Check sheet for the modelled part. Datum: model origin and axes. Units: mm. Face numbers are marked on the shaded views. A direction names the side the tool comes from. Give positions to 0.01 mm unless a question says otherwise; leave off trailing zeros. Write each loop counter-clockwise with the first axis right and the second up, starting at its lowest first coordinate (ties: lowest second). Pieces come first, ordered by that corner, then holes. Notation, with made-up numbers: M 22.25,63 L 30.25,63 A28 ccw 30.25,84 Z; hole C -36,35 d4. An arc over 180 degrees is marked long. Write item = value, one per line. Start each with the question number.
1) Sectioned sample at B-B, the plane x = 0. Record the cut outline in (y, z).
2) Draft check along Z on the marked faces 6, 7, 8 and 9. Enter one of: pulls with the +Z half, pulls with the -Z half, needs draft (parallel to the pull), parting line crosses it, or undercut.
3) Set-up check for the marked faces 1, 2, 3, 4 and 5: record each of +Z, -Z, +X, -X, +Y, -Y from which the full face is reachable in a straight line by a thin tool's end or side.
4) Gauge pin test, flat ends, axial feed: pin 1 (4.5 mm diameter, centred on y = -9.5, z = 89.5, fed in from -X); pin 2 (1.3 mm diameter, centred on y = 8.5, z = 89.5, fed in from +X); pin 3 (3 mm diameter, centred on y = 6.5, z = 90.5, fed in from +X). Record the tip position at first contact, or that the pin passes through.
5) Scan lines: L1, parallel to Y at x = -5.1, z = 92.5; L2, parallel to X at y = -10, z = 92.25; L3, parallel to Y at x = 0.5, z = 95. Record each from-to range of solid material in increasing order.
6) Sectioned sample at A-A, the plane y = 8. Record the cut outline in (x, z).
7) Sectioned sample at C-C, the plane z = 92.5. Count the separate pieces of the cut face and the enclosed holes in it, then the cut area to 3 significant figures.
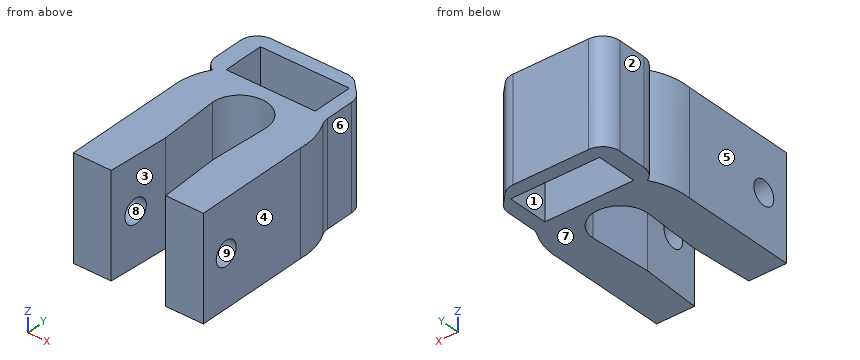
from build123d import *

# Parameters (mm, degrees)
CLIP_DEPTH          = 15
SKETCH7_R           = 1.75
CUT_EXTRUDE4_DEPTH  = 19.812
SKETCH8_W           = 17.539999972
SKETCH8_H           = 9.000000002
BOSS_EXTRUDE1_DEPTH = 15
SKETCH10_W          = 13
SKETCH10_H          = 6
CUT_EXTRUDE5_DEPTH  = 15
CHAMFER2_SIZE       = 3
FILLET1_R           = 2.5


with BuildPart() as part:
    # Sketch1 → Clip (new body)
    with BuildSketch(Plane(origin=(0, -100, 100), x_dir=(1, 0, 0), z_dir=(0, 0, -1))):
        with BuildLine():
            Line((-3.447825682, -91.120916541), (-3.96875, -100))
            ThreePointArc((-3.96875, -100), (0, -103.96875), (3.96875, -100))
            Line((3.96875, -100), (3.447825682, -91.120916541))
            Line((3.447825682, -91.120916541), (3.96875, -82.230916541))
            Line((3.96875, -82.230916541), (9.496072463, -82.230916541))
            Line((9.496072463, -82.230916541), (9.496072463, -99.258223228))
            ThreePointArc((9.496072463, -99.258223228), (0, -109.525), (-9.496072463, -99.258223228))
            Line((-9.496072463, -99.258223228), (-9.496072463, -82.230916541))
            Line((-9.496072463, -82.230916541), (-3.96875, -82.230916541))
            Line((-3.96875, -82.230916541), (-3.447825682, -91.120916541))
        make_face()
    extrude(amount=CLIP_DEPTH)

    # Sketch7 → Cut-Extrude4 (cut)
    with BuildSketch(Plane.ZY.offset(9.496072463)):
        with Locations(Location((92.5, -13.769083459, 0), (0, 0, 270))):
            Circle(SKETCH7_R)
    extrude(amount=-CUT_EXTRUDE4_DEPTH, mode=Mode.SUBTRACT)

    # Sketch8 → Boss-Extrude1 (add)
    with BuildSketch(Plane.XY.offset(100)):
        with Locations((-0.726072477, 9.499999907)):
            Rectangle(SKETCH8_W, SKETCH8_H)
    extrude(amount=-BOSS_EXTRUDE1_DEPTH)

    # Sketch10 → Cut-Extrude5 (cut)
    with BuildSketch(Plane(origin=(0, 0, 85), x_dir=(-1, 0, 0), z_dir=(0, 0, -1))):
        with Locations((0.456072491, 8.999999876)):
            Rectangle(SKETCH10_W, SKETCH10_H)
    extrude(amount=-CUT_EXTRUDE5_DEPTH, mode=Mode.SUBTRACT)

    # Chamfer2
    chamfer2_edges = [part.edges().sort_by_distance(p)[0] for p in [
        (8.043927509, 13.999999908, 92.5),
    ]]
    chamfer(chamfer2_edges, length=CHAMFER2_SIZE)

    # Fillet1
    # the kernel refuses this fillet: 2.5 mm, written as the material it adds along each edge
    with BuildSketch(Plane(origin=(8.043927509, 5.101064127, 85), x_dir=(0, 1, 0), z_dir=(0, 0, 1))) as fillet1_piece_1:
        with BuildLine():
            CenterArc((0.68047699, -2.5), FILLET1_R, 90, 28.737235663)
            ThreePointArc((-0.521506611, -0.307915279), (-0.258305429, -0.158103532), (0, 0))
            Line((0, 0), (0.68047699, 0))
        make_face()
    extrude(amount=15)
    # the kernel refuses this fillet: 2.5 mm, written as the material it takes off along each edge
    with BuildSketch(Plane(origin=(-9.496072463, 13.999999908, 106.25), x_dir=(1, 0, 0), z_dir=(0, 0, -1))) as fillet1_2_piece_1:
        with BuildLine():
            CenterArc((FILLET1_R, FILLET1_R), FILLET1_R, 180, 90)
            Line((0, FILLET1_R), (0, 0))
            Line((0, 0), (FILLET1_R, 0))
        make_face()
    extrude(amount=27.5, mode=Mode.SUBTRACT)
    with BuildSketch(Plane(origin=(-9.496072463, 4.999999906, 105.598851266), x_dir=(0, 1, 0), z_dir=(0, 0, -1))) as fillet1_2_piece_2:
        with BuildLine():
            CenterArc((2.239540506, 2.5), FILLET1_R, 206.386538366, 63.613461634)
            Line((0, 1.388938201), (0, 0))
            Line((0, 0), (2.239540506, 0))
        make_face()
    extrude(amount=26.197702531, mode=Mode.SUBTRACT)
    with BuildSketch(Plane(origin=(5.043927509, 13.999999908, 102.588834765), x_dir=(-1, 0, 0), z_dir=(0, 0, -1)), Plane(origin=(8.043927509, 10.999999908, 102.588834765), x_dir=(-0.7071067811865475, 0.7071067811865475, 0), z_dir=(0, 0, -1))) as fillet1_2_piece_3:
        with BuildLine():
            CenterArc((FILLET1_R * 0.414213562373, -FILLET1_R), FILLET1_R, 90, 45)
            Line((-FILLET1_R * 0.292893218813, -FILLET1_R * 0.292893218813), (0, 0))
            Line((0, 0), (FILLET1_R * 0.414213562373, 0))
        make_face()
    extrude(amount=20.17766953, mode=Mode.SUBTRACT)


solid = part.part
Data:
q1.outline = M 3.97,85 L 6,85 L 6,100 L 3.97,100 Z; M 12,85 L 14,85 L 14,100 L 12,100 Z
q2.face_6 = needs draft
q2.face_7 = pulls with the -Z half
q2.face_8 = undercut
q2.face_9 = undercut
q3.face_1 = +Z, -Z
q3.face_2 = +Z, -Z, -X, +Y
q3.face_3 = +Z, -Z, -Y
q3.face_4 = +Z, -Z, +X, -Y
q3.face_5 = +Z, -Z, -X, -Y
q4.pin_1 = -9.5
q4.pin_2 = 8.04
q4.pin_3 = 8.17
q5.L1 = -17.77 to -15.52, -12.02 to 6, 12 to 14
q5.L2 = -9.5 to -3.51, 3.51 to 9.5
q5.L3 = 3.94 to 6, 12 to 14
q6.outline = M -9.5,85 L -6.96,85 L -6.96,100 L -9.5,100 Z; M 6.04,85 L 8.04,85 L 8.04,100 L 6.04,100 Z
q7.separate_pieces = 3
q7.enclosed_holes = 1
q7.area = 304 mm2
